Check sheet for the modelled part. Datum: model origin and axes. Units: mm. A direction names the side the tool comes from. Coordinates: 2 decimals unless noted, no trailing zeros. Write each loop counter-clockwise with the first axis right and the second up, starting at its lowest first coordinate (ties: lowest second). Pieces come first, ordered by that corner, then holes. Notation, with made-up numbers: (22, -14) - (37, -14) arc R26 cw to (37, 17) - close; hole circle Ø1 at (-21, 74.5). An arc over 180 degrees is marked (long way). Answer as CSV lines item,"result". Start each with the question number.
from build123d import *

# Parameters (mm, degrees)
F0_W     = 571.5
F0_H     = 304.8
F1_DEPTH = 12.7
F2_W     = 19.05
F2_H     = 63.5
F3_DEPTH = 285.75
F4_W     = 19.05
F4_H     = 63.5
F5_DEPTH = 266.7


with BuildPart() as f1:
    # F0 (on Top) → F1 (new body)
    with BuildSketch(Plane.XY):
        Rectangle(F0_W, F0_H)
    extrude(amount=F1_DEPTH)

    # F2 (on Right) → F3 (join, symmetric)
    with BuildSketch(Plane.YZ):
        with Locations((-142.875, -31.75)):
            Rectangle(F2_W, F2_H)
    extrude(amount=F3_DEPTH, both=True)

    # F4 (on Right) → F5 (join, symmetric)
    with BuildSketch(Plane.YZ):
        with Locations((142.875, -31.75)):
            Rectangle(F4_W, F4_H)
    extrude(amount=F5_DEPTH, both=True)


solid = f1.part
(1) Release check for a two-part mould opening along Y. For faces 6 (the face through (4, -133.35, -32)), 7 (the face through (4, -152.4, -26)), 8 (the face through (-285.75, -34.6, 0.2)) record: pulls with the +Y half, pulls with the -Y half, needs draft (parallel to the pull), parting line crosses it, or undercut.
(2) Cross-section at A-A on z = -38. Record the boundary of the cut face in (x, y), plus the area to 3 significant figures.
(3) Cross-section at B-B on x = -9. Record the boundary of the cut face in (y, z).
(4) Tool access check on faces 1 (the face through (266.7, 143, -31)), 2 (the face through (4, -143, -63.5)), 3 (the face through (285.75, -34.6, 0.2)), 4 (the face through (4, 133.35, -32)), 5 (the face through (-266.7, 143, -31)). Record the directions out of +Z, -Z, +X, -X, +Y, -Y that give a thin tool (end or side, any length) a straight path to the whole face; none if there is none.
(5) Material ranges on probe 1 along Y at (x, z) = (183.5, -60); probe 2 along Z at (x, y) = (234.5, 5), recorded low to high. Write a range as from..to.
(6) Go/stop test with flat-tipped pins: P1, Ø1, axis at x = -120.5, y = -91, coming from the -Z side; P2, Ø15, axis at y = 139.5, z = -33, coming from the -X side; P3, Ø5.5, axis at y = 139.5, z = -20, coming from the +X side. Record where each tip stops, or that it passes through.
(7) Cross-section at C-C on y = -124. Record the boundary of the cut face in (x, z).
Checked values:
1,face 6,"undercut"
1,face 7,"pulls with the -Y half"
1,face 8,"needs draft"
2,outline,"(-285.75, -152.4) - (285.75, -152.4) - (285.75, -133.35) - (-285.75, -133.35) - close; (-266.7, 133.35) - (266.7, 133.35) - (266.7, 152.4) - (-266.7, 152.4) - close"
2,area,"21,000 mm^2"
3,outline,"(-152.4, -63.5) - (-133.35, -63.5) - (-133.35, 0) - (133.35, 0) - (133.35, -63.5) - (152.4, -63.5) - (152.4, 12.7) - (-152.4, 12.7) - close"
4,face 1,"-Z, +X, +Y"
4,face 2,"-Z, +X, -X, +Y, -Y"
4,face 3,"+Z, -Z, +X, +Y, -Y"
4,face 4,"-Z, +X, -X"
4,face 5,"-Z, -X, +Y"
5,probe 1,"-152.4..-133.35, 133.35..152.4"
5,probe 2,"0..12.7"
6,P1,"z = 0"
6,P2,"x = -266.7"
6,P3,"x = 266.7"
7,outline,"(-285.75, 0) - (285.75, 0) - (285.75, 12.7) - (-285.75, 12.7) - close"
